Model file for the job. Use its own axes, mm. Face numbers are marked on the shaded views. A direction names the side the tool comes from. Coordinates: 2 decimals unless noted, no trailing zeros. Write each loop counter-clockwise with the first axis right and the second up, starting at its lowest first coordinate (ties: lowest second). Pieces come first, ordered by that corner, then holes.
Q1. Band-saw the part on B-B, the plane y = 1.5. State how many separate pieces and enclosed holes the cut face has, plus the area to 3 significant figures.
Q2. Drill centre lines: probe 1 along Z at (x, y) = (0, 1.75); probe 2 along X at (y, z) = (1.1, 0) (3 decimals); probe 3 along Z at (x, y) = (-16, -2). Where is each one in solid material? Low to high.
Q3. Pull direction X, two halves, no side cores. Call the marked faces 6, 7, 8 and 9: released by +X, released by -X, zero draft, split by the parting line, or undercut.
Q4. Which spindle directions (+Z, -Z, +X, -X, +Y, -Y) get a long thin tool onto all of the face, cutting with end or side? Do the marked faces 1, 2, 3, 4 and 5. Say none if no direction does.
Q5. Pin check, flat tips, straight feed: P1, Ø1.5, axis at x = -34.5, z = 13.5, coming from the +Y side (3 decimals); P2, Ø5, axis at x = 15, y = -1.5, coming from the -Z side; P3, Ø1.4, axis at x = -16, y = -2, coming from the -Z side. Stop position of each tip, or through.
Q6. Band-saw the part on D-D, the plane x = -35.5. Write the cut outline in (y, z) (3 decimals).
Q7. Band-saw the part on A-A, the plane x = 0. Write the cut outline in (y, z) (3 decimals).
Q8. Band-saw the part on C-C, the plane z = -30.48. Write the cut outline in (x, y) (3 decimals), plus the area to 3 significant figures.
from build123d import *

# Parameters (mm, degrees)
SKETCH1_R                    = 3.175
SKETCH1_R_2                  = 1.5875
BOSS_EXTRUDE1_DEPTH          = 3.175
CUT_EXTRUDE1_REACH           = 61.599
BOSS_EXTRUDE2_DEPTH          = 3.175
TAP_DRILL_FOR_10_HELICOIL2_D = 5.1054
FILLET1_R                    = 2.54
CUT_EXTRUDE2_REACH           = 61.146
SKETCH20_W                   = 20.32
SKETCH20_H                   = 6.35
SKETCH22_R                   = 11.5
CUT_EXTRUDE3_DEPTH           = 3
BOSS_EXTRUDE4_START          = 2.75
BOSS_EXTRUDE4_DEPTH          = 2.75


with BuildPart() as part:
    # Sketch1 → Boss-Extrude1 (new body)
    with BuildSketch(Plane(origin=(0, 0, 0), x_dir=(1, 0, 0), z_dir=(0, 1, 0))):
        with BuildLine():
            Line((-20.32, 25.4), (-15.875, 25.4))
            Line((-15.875, 25.4), (0, 38.1))
            Line((0, 38.1), (15.875, 25.4))
            Line((15.875, 25.4), (20.32, 25.4))
            ThreePointArc((20.32, 25.4), (45.72, 0), (20.32, -25.4))
            Line((20.32, -25.4), (20.32, -31.75))
            Line((20.32, -31.75), (-20.32, -31.75))
            Line((-20.32, -31.75), (-20.32, -25.4))
            ThreePointArc((-20.32, -25.4), (-45.72, 0), (-20.32, 25.4))
        make_face()
        with Locations(Location((20.32, 0, 0), (0, 0, 270))):
            Circle(SKETCH1_R, mode=Mode.SUBTRACT)
        with Locations(Location((7.62, 21.997045256, 0), (0, 0, 270))):
            Circle(SKETCH1_R_2, mode=Mode.SUBTRACT)
        with Locations(Location((-20.32, 0, 0), (0, 0, 270))):
            Circle(SKETCH1_R, mode=Mode.SUBTRACT)
        with Locations(Location((-7.62, 21.997045256, 0), (0, 0, 270))):
            Circle(SKETCH1_R_2, mode=Mode.SUBTRACT)
    extrude(amount=BOSS_EXTRUDE1_DEPTH)

    # Sketch7 → Cut-Extrude1 (cut, up to next)
    with BuildSketch(Plane(origin=(0, 3.175, 0), x_dir=(1, 0, 0), z_dir=(0, 1, 0)), mode=Mode.PRIVATE) as cut_extrude1_sk1:
        with BuildLine():
            Line((-42.317045256, 12.7), (-39.017488468, 10.795))
            ThreePointArc((-39.017488468, 10.795), (-31.115, 18.697488468), (-20.32, 21.59))
            Line((-20.32, 21.59), (-15.875, 21.59))
            Line((-15.875, 21.59), (-15.875, 25.008038208))
            ThreePointArc((-15.875, 25.008038208), (-18.088875897, 25.301819801), (-20.32, 25.4))
            ThreePointArc((-20.32, 25.4), (-33.02, 21.997045256), (-42.317045256, 12.7))
        make_face()
    cut_extrude1_tool1 = extrude(cut_extrude1_sk1.sketch, amount=-CUT_EXTRUDE1_REACH, mode=Mode.PRIVATE) & part.part
    # Sketch7 → Cut-Extrude1 (cut, up to next)
    with BuildSketch(Plane(origin=(0, 3.175, 0), x_dir=(1, 0, 0), z_dir=(0, 1, 0)), mode=Mode.PRIVATE) as cut_extrude1_sk2:
        with BuildLine():
            Line((-15.875, 25.4), (-20.32, 25.4))
            ThreePointArc((-20.32, 25.4), (-18.088875897, 25.301819801), (-15.875, 25.008038208))
            Line((-15.875, 25.008038208), (-15.875, 25.4))
        make_face()
    cut_extrude1_tool2 = extrude(cut_extrude1_sk2.sketch, amount=-CUT_EXTRUDE1_REACH, mode=Mode.PRIVATE) & part.part
    cut_extrude1_1 = cut_extrude1_tool1.solids().sort_by_distance((-29.568041, 3.175, -20.060943))[0]
    add(cut_extrude1_1, mode=Mode.SUBTRACT)
    cut_extrude1_2 = cut_extrude1_tool2.solids().sort_by_distance((-16.984528, 3.175, -25.282569))[0]
    add(cut_extrude1_2, mode=Mode.SUBTRACT)
    cut_extrude1 = cut_extrude1_1 + cut_extrude1_2  # Cut-Extrude1 as one shape, for the pattern or mirror that repeats it

    # Sketch9 → Boss-Extrude2 (add)
    with BuildSketch(Plane(origin=(0, 3.175, 0), x_dir=(1, 0, 0), z_dir=(0, 1, 0))):
        with BuildLine():
            ThreePointArc((-20.32, -21.59), (-39.017488468, -10.795), (-39.017488468, 10.795))
            Line((-39.017488468, 10.795), (-42.317045256, 12.7))
            ThreePointArc((-42.317045256, 12.7), (-42.317045256, -12.7), (-20.32, -25.4))
            Line((-20.32, -25.4), (-20.32, -31.75))
            Line((-20.32, -31.75), (-10.16, -31.75))
            Line((-10.16, -31.75), (-10.16, -25.4))
            Line((-10.16, -25.4), (0, -25.4))
            Line((0, -25.4), (0, -21.59))
            Line((0, -21.59), (-20.32, -21.59))
        make_face()
        Polygon((0, 25.4), (0, 38.1), (-5.08, 34.036), (-5.08, 25.4), align=None)
    boss_extrude2 = extrude(amount=BOSS_EXTRUDE2_DEPTH)

    # Mirror1: Cut-Extrude1, Boss-Extrude2 across plane
    add(cut_extrude1.mirror(Plane(origin=(0, 0, 0), x_dir=(0, 0, 1), z_dir=(1, 0, 0))), mode=Mode.SUBTRACT)
    add(boss_extrude2.mirror(Plane(origin=(0, 0, 0), x_dir=(0, 0, 1), z_dir=(1, 0, 0))))

    # Tap Drill for #10 Helicoil2 (through all)
    with Locations(Plane(origin=(0, 6.35, 0), x_dir=(1, 0, 0), z_dir=(0, 1, 0))):
        with Locations((-15.24, -26.67), (15.24, -26.67), (0, 30.48)):
            Hole(TAP_DRILL_FOR_10_HELICOIL2_D / 2)

    # Fillet1
    fillet1_edges = [part.edges().sort_by_distance(p)[0] for p in [
        (5.08, 4.7625, -25.4),
        (0, 3.175, -38.1),
        (-5.08, 4.7625, -25.4),
    ]]
    fillet(fillet1_edges, radius=FILLET1_R)

    # Sketch20 → Cut-Extrude2 (cut, up to next)
    with BuildSketch(Plane(origin=(0, 3.175, 0), x_dir=(1, 0, 0), z_dir=(0, 1, 0)), mode=Mode.PRIVATE) as cut_extrude2_sk1:
        with Locations((0, -28.575)):
            Rectangle(SKETCH20_W, SKETCH20_H)
    cut_extrude2_tool1 = extrude(cut_extrude2_sk1.sketch, amount=-CUT_EXTRUDE2_REACH, mode=Mode.PRIVATE) & part.part
    add(cut_extrude2_tool1.solids().sort_by_distance((0, 3.175, 28.575))[0], mode=Mode.SUBTRACT)

    # Sketch22 → Cut-Extrude3 (cut)
    with BuildSketch(Plane.XZ):
        with Locations(Location((-20.32, 0, 0), (0, 0, 270))):
            Circle(SKETCH22_R)
    extrude(amount=-CUT_EXTRUDE3_DEPTH, mode=Mode.SUBTRACT)

    # Sketch23 → Boss-Extrude4 (add)
    with BuildSketch(Plane.XZ.offset(BOSS_EXTRUDE4_START)):
        with BuildLine():
            Line((18.18, -2.3454264), (18.18, -12.75))
            ThreePointArc((18.18, -12.75), (16.715533906, -16.285533906), (13.18, -17.75))
            Line((13.18, -17.75), (-29.32, -17.75))
            ThreePointArc((-29.32, -17.75), (-32.855533906, -16.285533906), (-34.32, -12.75))
            Line((-34.32, -12.75), (-34.32, 12.75))
            ThreePointArc((-34.32, 12.75), (-32.855533906, 16.285533906), (-29.32, 17.75))
            Line((-29.32, 17.75), (13.18, 17.75))
            ThreePointArc((13.18, 17.75), (16.715533906, 16.285533906), (18.18, 12.75))
            Line((18.18, 12.75), (18.18, 2.3454264))
            ThreePointArc((18.18, 2.3454264), (17.145, 0), (18.18, -2.3454264))
        make_face()
        with BuildLine():
            Line((-29.32, 12.25), (9.68, 12.25))
            ThreePointArc((9.68, 12.25), (11.801320344, 11.371320344), (12.68, 9.25))
            Line((12.68, 9.25), (12.68, -9.25))
            ThreePointArc((12.68, -9.25), (11.801320344, -11.371320344), (9.68, -12.25))
            Line((9.68, -12.25), (-29.32, -12.25))
            ThreePointArc((-29.32, -12.25), (-31.441320344, -11.371320344), (-32.32, -9.25))
            Line((-32.32, -9.25), (-32.32, 9.25))
            ThreePointArc((-32.32, 9.25), (-31.441320344, 11.371320344), (-29.32, 12.25))
        make_face(mode=Mode.SUBTRACT)
    extrude(amount=-BOSS_EXTRUDE4_DEPTH)


solid = part.part
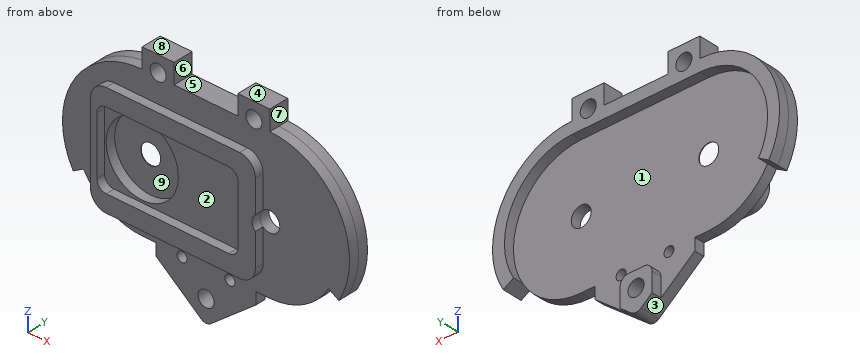
Answer sheet:
1. separate pieces: 1
1. enclosed holes: 7
1. area: 3,680 mm2
2. probe 1: z = -37.39 to -33.03, -27.93 to 25.4
2. probe 2: x = -45.72 to -31.82, -8.82 to 17.145, 23.495 to 45.72
2. probe 3: z = -17.75 to -12.25, 12.25 to 17.75
3. face 6: undercut
3. face 7: released by +X
3. face 8: zero draft
3. face 9: undercut
4. face 1: +Y
4. face 2: -Y
4. face 3: -Z, -X, +Y, -Y
4. face 4: +Z, +X, -X, +Y, -Y
4. face 5: +Z, +Y, -Y
5. P1: stops at y = 3.175
5. P2: stops at z = -27.7
5. P3: stops at z = -17.75
6. outline: (0, -15.352) - (3.175, -15.352) - (3.175, 15.352) - (6.35, 15.352) - (6.35, 20.365) - (0, 20.365) - close
7. outline: (-2.75, -17.75) - (0, -17.75) - (0, -27.927) - (6.35, -27.927) - (6.35, -25.4) - (3.175, -25.4) - (3.175, 21.59) - (6.35, 21.59) - (6.35, 25.4) - (0, 25.4) - (0, 17.75) - (-2.75, 17.75) - (-2.75, 12.25) - (0, 12.25) - (0, -12.25) - (-2.75, -12.25) - close; (0, -37.387) - (6.35, -37.387) - (6.35, -33.033) - (0, -33.033) - close
8. outline: (-9.525, 0) - (-2.553, 0) - (-2.553, 6.35) - (-5.08, 6.35) - (-5.08, 3.175) - (-9.525, 3.175) - close; (2.553, 0) - (9.525, 0) - (9.525, 3.175) - (5.08, 3.175) - (5.08, 6.35) - (2.553, 6.35) - close
8. area: 60.3 mm2
